```python
from build123d import *

# Parameters (mm, degrees)
SKETCH1_R           = 45
BOSS_EXTRUDE1_DEPTH = 4


with BuildPart() as part:
    # Sketch1 → Boss-Extrude1 (new body)
    with BuildSketch(Plane.XY):
        Circle(SKETCH1_R)
        with BuildLine():
            Line((-10.969996065, 35.702684582), (0, 11.06367001))
            Line((0, 11.06367001), (10.969996065, 35.702684582))
            ThreePointArc((10.969996065, 35.702684582), (0, 37.35), (-10.969996065, 35.702684582))
        make_face(mode=Mode.SUBTRACT)
        with BuildLine():
            Line((-10.969996065, -35.702684582), (0, -11.06367001))
            Line((0, -11.06367001), (10.969996065, -35.702684582))
            ThreePointArc((10.969996065, -35.702684582), (0, -37.35), (-10.969996065, -35.702684582))
        make_face(mode=Mode.SUBTRACT)
        with BuildLine():
            Line((-35.521960884, 11.54178474), (-15.191613619, -34.120922843))
            ThreePointArc((-15.191613619, -34.120922843), (-34.120922843, -15.191613619), (-35.521960884, 11.54178474))
        make_face(mode=Mode.SUBTRACT)
        with BuildLine():
            Line((-30.272016712, 21.877557089), (-12.728681992, -17.525417828))
            Line((-12.728681992, -17.525417828), (-5.426745524, -1.125))
            Line((-5.426745524, -1.125), (5.426745524, -1.125))
            Line((5.426745524, -1.125), (12.728681992, -17.525417828))
            Line((12.728681992, -17.525417828), (30.272016712, 21.877557089))
            ThreePointArc((30.272016712, 21.877557089), (25.248745429, 27.523142159), (19.191905184, 32.042054794))
            Line((19.191905184, 32.042054794), (5.426745524, 1.125))
            Line((5.426745524, 1.125), (-5.426745524, 1.125))
            Line((-5.426745524, 1.125), (-19.191905184, 32.042054794))
            ThreePointArc((-19.191905184, 32.042054794), (-25.248745429, 27.523142159), (-30.272016712, 21.877557089))
        make_face(mode=Mode.SUBTRACT)
        with BuildLine():
            Line((35.521960884, 11.54178474), (15.191613619, -34.120922843))
            ThreePointArc((15.191613619, -34.120922843), (34.120922843, -15.191613619), (35.521960884, 11.54178474))
        make_face(mode=Mode.SUBTRACT)
    extrude(amount=BOSS_EXTRUDE1_DEPTH)


solid = part.part
```
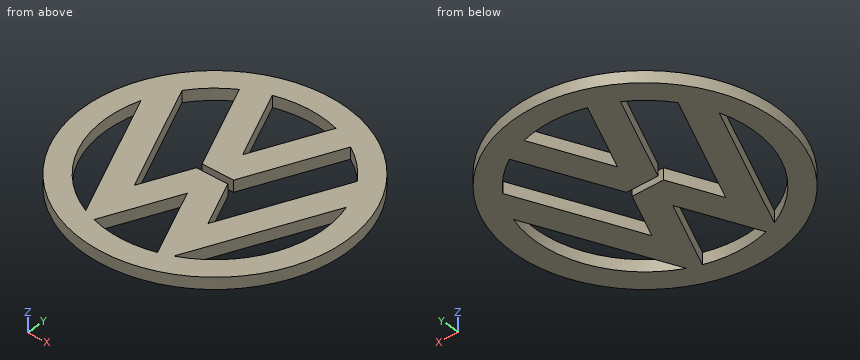
Here's how the part is built. I have some questions about the finished solid (model axes, mm). Give positions to 0.01 mm unless a question says otherwise; leave off trailing zeros. Loops run counter-clockwise (first coordinate to the right, second up) from the corner with the lowest first, then second, coordinate; pieces in that order, holes last. Notation, with made-up numbers: M 10,-28 L 57,-28 A24 ccw 57,-10 Z; hole C 22.5,65.5 d6. An arc over 180 degrees is marked long. Use one line per item in the form item = value. Start each with the question number.
Q1. Will these pins go through, and if not, where does the flat tip stop? pin 1 Ø1 at (y, z) = (-7, 3.5) entering from -X; pin 2 Ø1.5 at (y, z) = (13.5, 1.5) entering from +X; pin 3 Ø1 at (x, z) = (21, 0.5) entering from -Y.
Q2. I need wall thicknesses on line 1 along Y through (x, z) = (5, 1.2) (3 decimals); line 2 along X through (y, z) = (27.5, 3.85); line 3 along Y through (x, z) = (-1.5, 1.6) (3 decimals). Which ranges of each line are inside material? Lowest first, please.
Q3. If we section it at A-A (z = 2.45): Write out the boundary of the cut face in (x, y) (3 decimals), then the cut area to 3 significant figures.
Q4. If we section it at C-C (y = 0): Write out the boundary of the cut face in (x, z), then the cut area to 3 significant figures.
Q5. If we section it at D-D (y = -10): Write out the boundary of the cut face in (x, z).
Q6. If we section it at B-B (x = 34): Write out the boundary of the cut face in (y, z).
Taken from the geometry:
q1.pin_1 = -44.53
q1.pin_2 = 43.16
q1.pin_3 = -40.06
q2.line_1 = -44.721 to -37.014, -22.294 to -1.125, 1.125 to 22.294, 37.014 to 44.721
q2.line_2 = -35.62 to -25.27, -17.17 to -7.32, 7.32 to 17.17, 25.27 to 35.62
q2.line_3 = -44.975 to -37.32, -14.433 to -1.125, 1.125 to 14.433, 37.32 to 44.975
q3.outline = C 0,0 d90; hole M -35.522,11.542 A37.35 ccw -15.192,-34.121 Z; hole M -30.272,21.878 L -12.729,-17.525 L -5.427,-1.125 L 5.427,-1.125 L 12.729,-17.525 L 30.272,21.878 A37.35 ccw 19.192,32.042 L 5.427,1.125 L -5.427,1.125 L -19.192,32.042 A37.35 ccw Z; hole M -10.97,-35.703 A37.35 ccw 10.97,-35.703 L 0,-11.064 Z; hole M -10.97,35.703 L 0,11.064 L 10.97,35.703 A37.35 ccw Z; hole M 15.192,-34.121 A37.35 ccw 35.522,11.542 Z
q3.area = 3,960 mm^2
q4.outline = M -45,0 L -37.35,0 L -37.35,4 L -45,4 Z; M -30.38,0 L -20.53,0 L -20.53,4 L -30.38,4 Z; M 20.53,0 L 30.38,0 L 30.38,4 L 20.53,4 Z; M 37.35,0 L 45,0 L 45,4 L 37.35,4 Z
q4.area = 140 mm^2
q5.outline = M -43.87,0 L -35.99,0 L -35.99,4 L -43.87,4 Z; M -25.93,0 L -16.08,0 L -16.08,4 L -25.93,4 Z; M -9.38,0 L 9.38,0 L 9.38,4 L -9.38,4 Z; M 16.08,0 L 25.93,0 L 25.93,4 L 16.08,4 Z; M 35.99,0 L 43.87,0 L 43.87,4 L 35.99,4 Z
q6.outline = M -29.48,0 L -15.46,0 L -15.46,4 L -29.48,4 Z; M 8.12,0 L 29.48,0 L 29.48,4 L 8.12,4 Z
